Source: CAD feature listing. Evaluate the final solid. Frame: model axes, mm. A direction names the side the tool comes from. Give positions to 0.01 mm unless a question says otherwise; leave off trailing zeros. Write each loop counter-clockwise with the first axis right and the second up, starting at its lowest first coordinate (ties: lowest second). Pieces come first, ordered by that corner, then holes. Notation, with made-up numbers: M -38,-15 L -31,-15 A34 ccw -31,18 Z; hole C 66.25,-10 d2. An arc over 180 degrees is marked long. Return JSON: item names as keys, results as strings.
```python
from build123d import *

# Parameters (mm, degrees)
SKETCH1_W           = 80
SKETCH1_H           = 120
BOSS_EXTRUDE1_DEPTH = 100
SKETCH2_R           = 2.25
SKETCH2_R_2         = 1.5
BOSS_EXTRUDE2_DEPTH = 5
FILLET1_R           = 1


with BuildPart() as part:
    # Sketch1 → Boss-Extrude1 (new body)
    with BuildSketch(Plane(origin=(0, 0, 0), x_dir=(1, 0, 0), z_dir=(0, 1, 0))):
        Rectangle(SKETCH1_W, SKETCH1_H)
    extrude(amount=BOSS_EXTRUDE1_DEPTH)

    # Sketch2 → Boss-Extrude2 (add)
    with BuildSketch(Plane(origin=(0, 100, 0), x_dir=(1, 0, 0), z_dir=(0, 1, 0))):
        with Locations((0, 40)):
            Circle(SKETCH2_R)
        with Locations((0, 40)):
            Circle(SKETCH2_R_2, mode=Mode.SUBTRACT)
    extrude(amount=BOSS_EXTRUDE2_DEPTH)

    # Fillet1
    fillet1_edges = [part.edges().sort_by_distance(p)[0] for p in [
        (-40, 100, 0),
        (0, 100, 60),
        (40, 100, 0),
        (0, 100, -60),
    ]]
    fillet(fillet1_edges, radius=FILLET1_R)


solid = part.part
```
1) Cut plane C-C, the plane z = 26.5. Return the cut outline in (x, y), then the cut area to 3 significant figures.
Numbers:
{"outline": "M -40,0 L 40,0 L 40,99 A1 ccw 39,100 L -39,100 A1 ccw -40,99 Z", "area": "8,000 mm²"}
2) Set-up query: faces 4 (the face through (0, 100, -40)), 5 (the face through (-1, 49, -60)). Return all of +Z, -Z, +X, -X, +Y, -Y with unobstructed straight access to the full face (end or side cutting, diameter ignored); none if empty.
Numbers:
{"face 4": "+Y", "face 5": "-Z, +X, -X, +Y, -Y"}
3) Contact query for a flat-ended pin moving along its axis: pin 1 Ø23.5 at (x, z) = (0, -3.5) entering from +Y. Output: stop coordinate, or through.
Numbers:
{"pin 1": "stops at y = 100"}
4) Cut plane A-A, the plane z = -40. Return the cut outline in (x, y), then the cut area to 3 significant figures.
Numbers:
{"outline": "M -40,0 L 40,0 L 40,99 A1 ccw 39,100 L 2.25,100 L 2.25,105 L 1.5,105 L 1.5,100 L -1.5,100 L -1.5,105 L -2.25,105 L -2.25,100 L -39,100 A1 ccw -40,99 Z", "area": "8,010 mm²"}
5) Line query: line 1 (Z direction, x = 0, y = 102.5); line 2 (X direction, y = 103.95, z = -40); line 3 (Y direction, x = 17, z = 10.5). Output: solid intervals per line, ascending. Write a range as [from, to].
Numbers:
{"line 1": "z = [-42.25, -41.5], [-38.5, -37.75]", "line 2": "x = [-2.25, -1.5], [1.5, 2.25]", "line 3": "y = [0, 100]"}
6) Cut plane B-B, the plane x = 0. Return the cut outline in (y, z), then the cut area to 3 significant figures.
Numbers:
{"outline": "M 0,-60 L 99,-60 A1 ccw 100,-59 L 100,-42.25 L 105,-42.25 L 105,-41.5 L 100,-41.5 L 100,-38.5 L 105,-38.5 L 105,-37.75 L 100,-37.75 L 100,59 A1 ccw 99,60 L 0,60 Z", "area": "12,000 mm²"}
7) Draft query along Z for faces 1 (the face through (-40, 49, 1)), 2 (the face through (-0.325, 102.465, -38.536)), 3 (the face through (-1, 49, 60)). Return one class per face: released by +Z, released by -Z, zero draft, split by the parting line, or undercut.
Numbers:
{"face 1": "zero draft", "face 2": "undercut", "face 3": "released by +Z"}
8) Cut plane D-D, the plane x = -15.5. Return the cut outline in (y, z).
Numbers:
{"outline": "M 0,-60 L 99,-60 A1 ccw 100,-59 L 100,59 A1 ccw 99,60 L 0,60 Z"}
